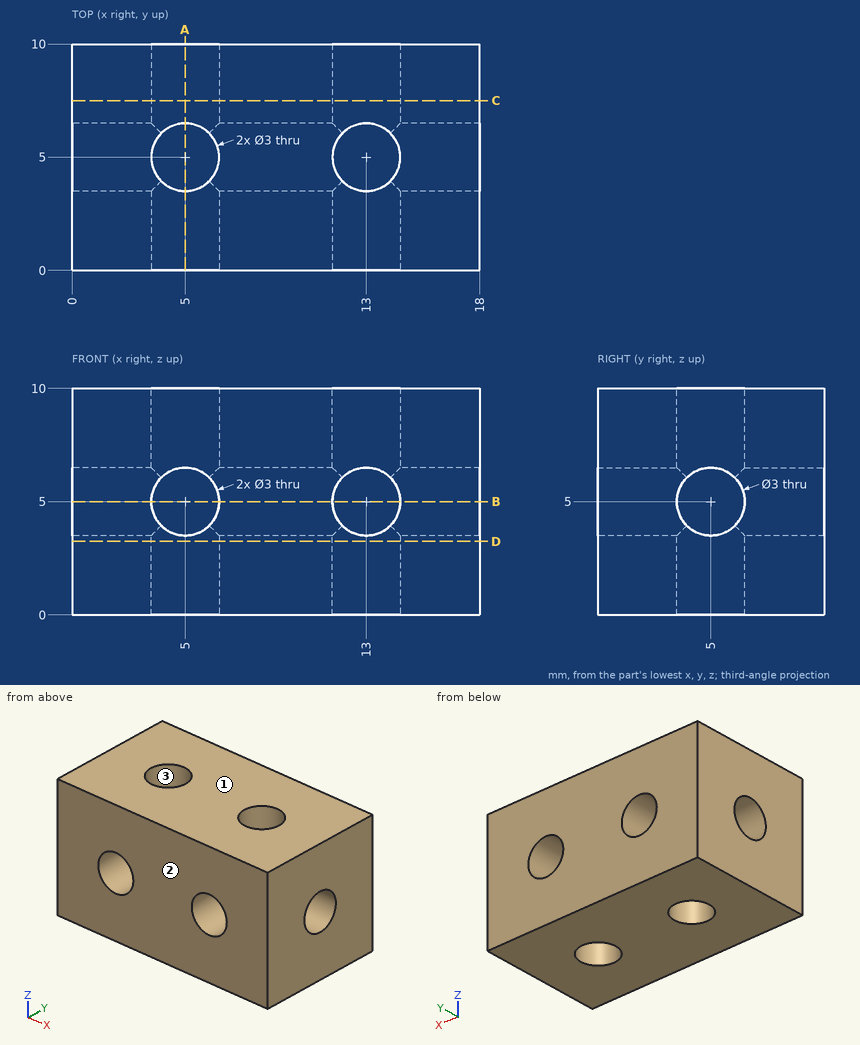
Input: dimensioned drawing with shaded views. Units: mm. Origin: part minimum x, y, z. Coordinates: 2 decimals unless noted, no trailing zeros. Order: outer loops, then holes, each group sorted by start corner. A loop starts at its lowest first (then second) coordinate and runs counter-clockwise, first axis right, second up.
(1) First-contact query: pin 1 (2.5 mm diameter, centred on x = 13, y = 5, fed in from -Z). Flat tip, straight axial feed; report the tip coordinate or a pass-through.
(2) Section query C-C (y = 7.5). Return the cut outline in (x, z).
(3) Section query B-B (z = 5). Return the cut outline in (x, y).
(4) Draft query along Y for the marked faces 1, 2 and 3. Return one class per face: pulls with the +Y half, pulls with the -Y half, needs draft (parallel to the pull), parting line crosses it, or undercut.
(5) Material intervals for probe 1 along X at (y, z) = (5, 3); probe 2 along X at (y, z) = (4.5, 6.5); probe 3 along Z at (x, y) = (2.25, 5), sorted ascending.
(6) Section query A-A (x = 5). Return the cut outline in (y, z), plus the area to 3 significant figures.
Solution:
1. pin 1: passes through
2. outline: (0, 0) - (18, 0) - (18, 10) - (0, 10) - close; hole circle Ø3 at (5, 5); hole circle Ø3 at (13, 5)
3. outline: (0, 0) - (3.5, 0) - (3.5, 3.5) - (0, 3.5) - close; (0, 6.5) - (3.5, 6.5) - (3.5, 10) - (0, 10) - close; (6.5, 0) - (11.5, 0) - (11.5, 3.5) - (6.5, 3.5) - close; (6.5, 6.5) - (11.5, 6.5) - (11.5, 10) - (6.5, 10) - close; (14.5, 0) - (18, 0) - (18, 3.5) - (14.5, 3.5) - close; (14.5, 6.5) - (18, 6.5) - (18, 10) - (14.5, 10) - close
4. face 1: needs draft
4. face 2: pulls with the -Y half
4. face 3: undercut
5. probe 1: x = 0 to 3.5, 6.5 to 11.5, 14.5 to 18
5. probe 2: x = 0 to 3.59, 6.41 to 11.59, 14.41 to 18
5. probe 3: z = 0 to 3.5, 6.5 to 10
6. outline: (0, 0) - (3.5, 0) - (3.5, 3.5) - (0, 3.5) - close; (0, 6.5) - (3.5, 6.5) - (3.5, 10) - (0, 10) - close; (6.5, 0) - (10, 0) - (10, 3.5) - (6.5, 3.5) - close; (6.5, 6.5) - (10, 6.5) - (10, 10) - (6.5, 10) - close
6. area: 49.0 mm2
